Work out the finished part from the listing and answer in its coordinate system (mm). A direction names the side the tool comes from. Coordinates: 2 decimals unless noted, no trailing zeros. Loops run counter-clockwise (first coordinate to the right, second up) from the corner with the lowest first, then second, coordinate; pieces in that order, holes last. Notation, with made-up numbers: M 61,28 L 89,28 A29 ccw 89,48 Z; hole C 64.25,27.5 d8. An arc over 180 degrees is marked long. Write each question's results on one line, items separated by ' | '.
```python
from build123d import *

# Parameters (mm, degrees)
SKETCH2_R           = 2.65
BOSS_EXTRUDE1_DEPTH = 2
CUT_EXTRUDE1_DEPTH  = 1.5


with BuildPart() as part:
    # Sketch2 → Boss-Extrude1 (new body)
    with BuildSketch(Plane(origin=(0, 0, 0), x_dir=(1, 0, 0), z_dir=(0, 1, 0))):
        with BuildLine():
            Line((-15.984695958, -228.591802117), (-17.334483725, -247.89466649))
            ThreePointArc((-17.334483725, -247.89466649), (0, -248.5), (17.334483725, -247.89466649))
            Line((17.334483725, -247.89466649), (15.984695958, -228.591802117))
            ThreePointArc((15.984695958, -228.591802117), (0, -229.15), (-15.984695958, -228.591802117))
        make_face()
        with Locations(Location((0, -236.25, 0), (0, 0, 270))):
            Circle(SKETCH2_R, mode=Mode.SUBTRACT)
    extrude(amount=BOSS_EXTRUDE1_DEPTH)

    # Sketch3 → Cut-Extrude1 (cut)
    with BuildSketch(Plane(origin=(0, 0, 0), x_dir=(1, 0, 0), z_dir=(0, 1, 0))):
        Polygon((0, -240.406921938), (3.6, -238.328460969), (3.6, -234.171539031), (0, -232.093078062), (-3.6, -234.171539031), (-3.6, -238.328460969), align=None)
    extrude(amount=CUT_EXTRUDE1_DEPTH, mode=Mode.SUBTRACT)


solid = part.part
```
1) Which of the six approach directions +Z, -Z, +X, -X, +Y, -Y give full straight-line access (tool end or side, diameter ignored) to faces 4 (the face through (3.6, 1, 236)), 5 (the face through (0.22, 0.99, 229.15))?
Check result:
face 4: -Y | face 5: -Z, +Y, -Y
2) Find section D-D, the plane z = 244. Give the vertices of the cut face in (x, y), and give its area (3 significant figures).
Check result:
outline: M -17.06,0 L 17.06,0 L 17.06,2 L -17.06,2 Z | area: 68.2 mm^2
3) Find section A-A, the plane z = 237.75. Give the vertices of the cut face in (x, y).
Check result:
outline: M -16.63,0 L -3.6,0 L -3.6,1.5 L -2.18,1.5 L -2.18,2 L -16.63,2 Z; M 2.18,1.5 L 3.6,1.5 L 3.6,0 L 16.63,0 L 16.63,2 L 2.18,2 Z
4) Find section B-B, the plane y = 0.4. Give the vertices of the cut face in (x, z), and give its area (3 significant figures).
Check result:
outline: M -17.33,247.89 L -15.98,228.59 A229.15 cw 15.98,228.59 L 17.33,247.89 A248.5 ccw Z; hole M -3.6,234.17 L 0,232.09 L 3.6,234.17 L 3.6,238.33 L 0,240.41 L -3.6,238.33 Z | area: 600 mm^2
5) For a pull along X with two mould halves and no side action, classify faces 1 (the face through (-0.2, 1, 248.5)), 2 (the face through (-1.83, 0.74, 239.35)), 3 (the face through (16.67, 0.99, 238.38)) as released by +X, released by -X, zero draft, split by the parting line, or undercut.
Check result:
face 1: split by the parting line | face 2: undercut | face 3: released by +X
6) Find section C-C, the plane x = 2. Give the vertices of the cut face in (y, z).
Check result:
outline: M 0,229.14 L 2,229.14 L 2,234.51 L 1.5,234.51 L 1.5,233.25 L 0,233.25 Z; M 0,239.25 L 1.5,239.25 L 1.5,237.99 L 2,237.99 L 2,248.49 L 0,248.49 Z
7) Given pin 1 Ø0.8 at (y, z) = (0.5, 236.5) entering from +X; pin 2 Ø1 at (x, y) = (7, 1.5) entering from +Z (3 decimals); pin 3 Ø0.8 at (y, z) = (0.5, 237) entering from -X, each flat-ended and moving along its own axis, determine where each tip first touches the part or whether it passes through.
Check result:
pin 1: x = 16.57 | pin 2: z = 248.415 | pin 3: x = -16.6
8) Straight lines are drawn through the part: probe 1 along X at (y, z) = (1.7, 234.5); probe 2 along Z at (x, y) = (-3, 0.2); probe 3 along X at (y, z) = (1.85, 236.25). For each, find the intervals that lie inside material, in ascending order. Write a range as [from, to].
Check result:
probe 1: [-16.4, -1.99], [1.99, 16.4] | probe 2: [229.13, 233.83], [238.67, 248.48] | probe 3: [-16.52, -2.65], [2.65, 16.52]
